Source: three-view drawing plus pictorial views. Frame: mm from the lowest corner of the part. Give positions to 0.01 mm unless a question says otherwise; leave off trailing zeros. Order: outer loops, then holes, each group sorted by start corner. A loop starts at its lowest first (then second) coordinate and runs counter-clockwise, first axis right, second up.
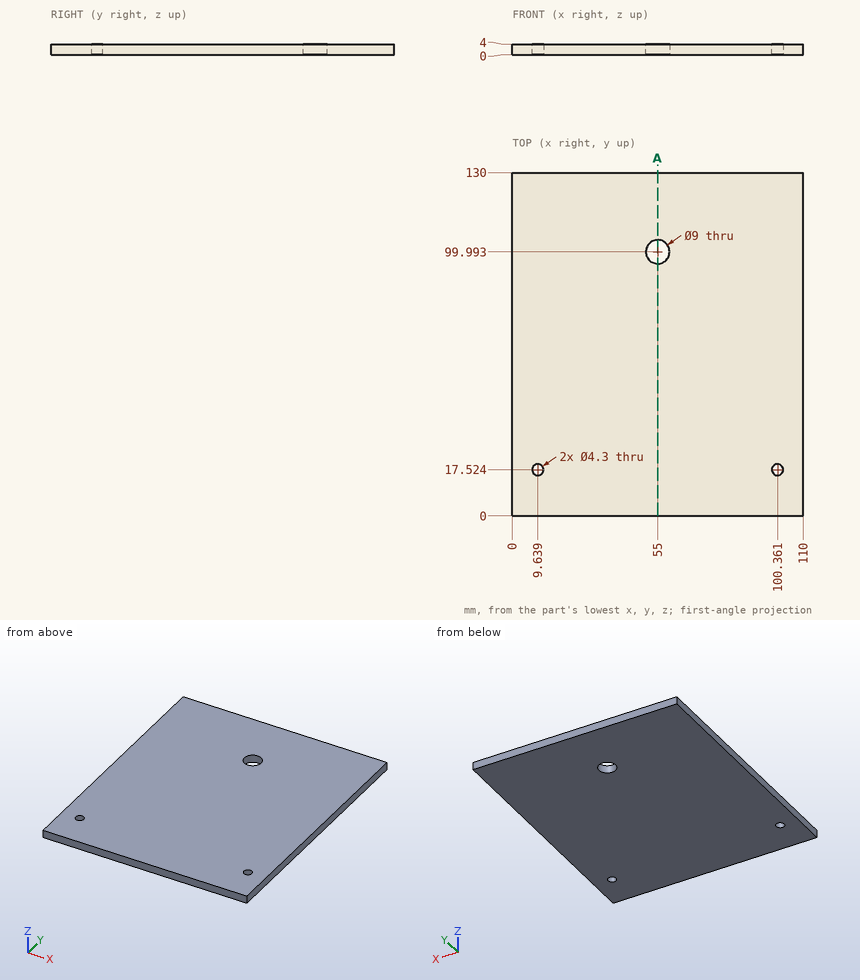
1) First-contact query: pin 1 Ø2.5 at (x, y) = (100.36, 17.52) entering from -Z; pin 2 Ø5.5 at (x, y) = (9.64, 17.52) entering from -Z. Flat tips, straight axial feed; report the tip coordinate or a pass-through.
Checks:
pin 1: passes through
pin 2: stops at z = 0
2) Section query A-A on x = 55. Output: boundary loops of the cut face in (y, z), and give its area (3 significant figures).
Checks:
outline: (0, 0) - (95.49, 0) - (95.49, 4) - (0, 4) - close; (104.49, 0) - (130, 0) - (130, 4) - (104.49, 4) - close
area: 484 mm2
3) Ray query, L1, parallel to X at y = 18.5, z = 2.3 (1 decimal); L2, parallel to Y at x = 10, z = 1.65 (1 decimal); L3, parallel to Y at x = 9, z = 2.25. Return the intervals inside material, ascending.
Checks:
L1: x = 0 to 7.7, 11.6 to 98.4, 102.3 to 110
L2: y = 0 to 15.4, 19.6 to 130
L3: y = 0 to 15.47, 19.58 to 130
